```python
from build123d import *

# Parameters (mm, degrees)
SKETCH1_R           = 2.9845
BOSS_EXTRUDE1_DEPTH = 6.35
CUT_EXTRUDE1_DEPTH  = 7.35
FILLET1_R           = 25.4
FILLET2_R           = 6.35
FILLET3_R           = 1.905
FILLET4_R           = 2.54


with BuildPart() as part:
    # Sketch1 → Boss-Extrude1 (new body)
    with BuildSketch(Plane(origin=(0, 0, 0), x_dir=(1, 0, 0), z_dir=(0, 1, 0))):
        with BuildLine():
            Line((7.682408093, 3.020865917), (5.624249106, 8.255))
            Line((5.624249106, 8.255), (0, 8.255))
            ThreePointArc((0, 8.255), (-6.323696878, 5.306211718), (-8.129588001, -1.433465707))
            Line((-8.129588001, -1.433465707), (-1.513592432, -38.954641096))
            ThreePointArc((-1.513592432, -38.954641096), (33.306036144, -50.744311292), (69.85, -54.737))
            ThreePointArc((69.85, -54.737), (72.817340251, -54.71098351), (75.783768162, -54.632942041))
            Line((75.783768162, -54.632942041), (25.4, -42.037))
            Line((25.4, -42.037), (7.682408093, 3.020865917))
        make_face()
        Circle(SKETCH1_R, mode=Mode.SUBTRACT)
    extrude(amount=BOSS_EXTRUDE1_DEPTH)

    # Sketch2 → Cut-Extrude1 (cut, through all)
    with BuildSketch(Plane(origin=(0, 6.35, 0), x_dir=(1, 0, 0), z_dir=(0, 1, 0))):
        Polygon((4.007338902, -34.519082642), (18.219473265, -41.128490063), (4.543923357, -6.35), (-0.959630389, -6.35), align=None)
    extrude(amount=-CUT_EXTRUDE1_DEPTH, mode=Mode.SUBTRACT)

    # Fillet1
    fillet1_edges = [part.edges().sort_by_distance(p)[0] for p in [
        (25.4, 3.175, 42.037),
    ]]
    fillet(fillet1_edges, radius=FILLET1_R)

    # Fillet2
    fillet2_edges = [part.edges().sort_by_distance(p)[0] for p in [
        (-1.513592432, 3.175, 38.954641096),
    ]]
    fillet(fillet2_edges, radius=FILLET2_R)

    # Fillet3
    fillet3_edges = [part.edges().sort_by_distance(p)[0] for p in [
        (-0.959630389, 3.175, 6.35),
        (4.543923357, 3.175, 6.35),
        (18.219473265, 3.175, 41.128490063),
        (4.007338902, 3.175, 34.519082642),
    ]]
    fillet(fillet3_edges, radius=FILLET3_R)

    # Fillet4
    fillet4_edges = [part.edges().sort_by_distance(p)[0] for p in [
        (5.624249106, 3.175, -8.255),
    ]]
    fillet(fillet4_edges, radius=FILLET4_R)


solid = part.part
```
Model file for the job. Use its own axes, mm. A direction names the side the tool comes from. Give positions to 0.01 mm unless a question says otherwise; leave off trailing zeros. Order: outer loops, then holes, each group sorted by start corner. A loop starts at its lowest first (then second) coordinate and runs counter-clockwise, first axis right, second up.
1) Mould opens along X. For faces 3 (the cylindrical face through (-0.647, 3.131, 2.914)), 4 (the cylindrical face through (-6.26, 3.13, -5.38)), 5 (the cylindrical face through (27.365, 3.219, 39.542)) say: +X half, -X half, draft (parallel to the pull), parting line (faces both ways), or undercut.
2) Saw through at A-A, the plane y = 5.5. Count the separate pieces of the cut face and the enclosed holes in it, then the cut area to 3 significant figures.
3) Pin check, flat tips, straight feed: pin 1 (1.5 mm diameter, centred on y = 1.5, z = 33, fed in from -X); pin 2 (2 mm diameter, centred on y = 3.5, z = 0.5, fed in from +X); pin 3 (1 mm diameter, centred on x = 2.5, y = 3, fed in from +Z); pin 4 (9.5 mm diameter, centred on x = 0, z = 0, fed in from -Y). Stop position of each tip, or through.
4) Wall check: probe 1 along X at (y, z) = (3, 0) (1 decimal); probe 2 along X at (y, z) = (1, 19.5); probe 3 along Z at (x, y) = (56.5, 4). Give the ranges that are in metal, low to high.
5) 3-axis set-ups, long thin cutter, end or side, ignore diameter. For faces 1 (the flat face through (1.604, 3.219, 20.889)), 2 (the flat face through (15, 6.35, 28)): which of +Z, -Z, +X, -X, +Y, -Y reach the whole face in a straight line?
6) Saw through at C-C, the plane x = 49. Write the cut outline in (y, z), then the cut area to 3 significant figures.
7) Saw through at B-B, the plane z = 26. Write the cut outline in (x, y).
Computed:
1. face 3: undercut
1. face 4: -X half
1. face 5: +X half
2. separate pieces: 1
2. enclosed holes: 2
2. area: 1,050 mm2
3. pin 1: stops at x = -2.7
3. pin 2: stops at x = 9.46
3. pin 3: stops at z = 40.97
3. pin 4: stops at y = 0
4. probe 1: x = -8.3 to -3, 3 to 8.9
4. probe 2: x = -4.94 to 1.36, 9.71 to 16.54
4. probe 3: z = 49.81 to 54.21
5. face 1: +Y, -Y
5. face 2: +Z, -Z, +X, -X, +Y
6. outline: (0, 47.94) - (6.35, 47.94) - (6.35, 53.45) - (0, 53.45) - close
6. area: 35.0 mm2
7. outline: (-3.8, 0) - (2.51, 0) - (2.51, 6.35) - (-3.8, 6.35) - close; (12.27, 0) - (19.09, 0) - (19.09, 6.35) - (12.27, 6.35) - close
